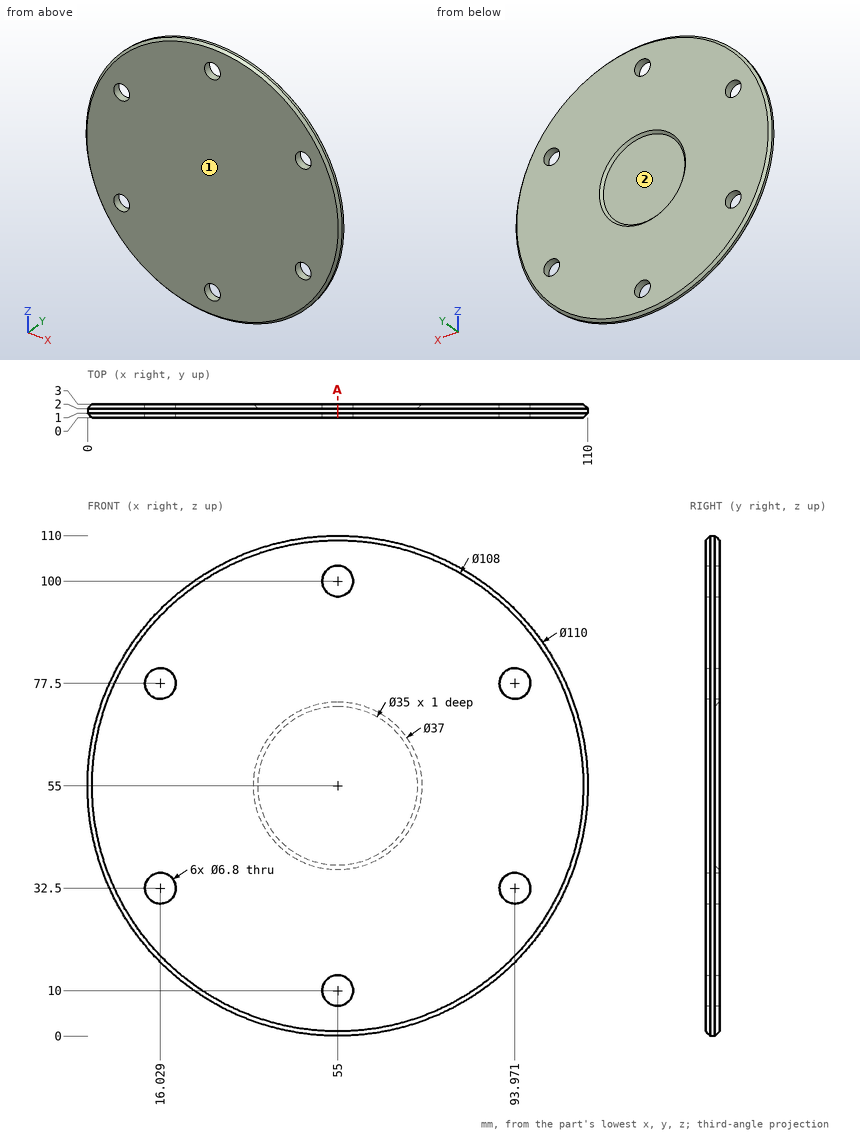
Part print with two shaded views. Sizes in mm from the minimum x, y, z corner. Give positions to 0.01 mm unless a question says otherwise; leave off trailing zeros. Use one line per item in the form item = value.
1) Drop flat-ended pins along their axis: pin 1 (6 mm diameter, centred on x = 96, z = 97.5, fed in from -Y); pin 2 (1 mm diameter, centred on x = 89, y = 1, fed in from +Z). Give the stop position or say it passes through.
Calculated:
pin_1 = through
pin_2 = 98.62
2) Probe probe 1 along X at (y, z) = (0.9, 32.5); probe 2 along Z at (x, y) = (92, 0.25) (1 decimal); probe 3 along Z at (x, y) = (16, 1.15). List the from-to ranges inside material, lowest first.
Calculated:
probe_1 = 4.92 to 12.63, 19.43 to 90.57, 97.37 to 105.08
probe_2 = 15.3 to 29.7, 35.3 to 74.7, 80.3 to 94.7
probe_3 = 16.22 to 29.1, 35.9 to 74.1, 80.9 to 93.78
3) Two-plate mould, pull along Z, no slides. Class the marked faces 1 and 2: released by +Z, released by -Z, zero draft, split by the parting line, or undercut.
Calculated:
face_1 = zero draft
face_2 = undercut
4) Saw through at A-A (x = 55). State how many separate pieces and enclosed holes the cut face has, plus the area to 3 significant figures.
Calculated:
separate_pieces = 3
enclosed_holes = 0
area = 251 mm2
